For this review, use the dimensioned drawing (mm, ordinates from the lowest corner) and the shaded views. Coordinates: 2 decimals unless noted, no trailing zeros. Order: outer loops, then holes, each group sorted by start corner. A loop starts at its lowest first (then second) coordinate and runs counter-clockwise, first axis right, second up. Notation, with made-up numbers: (8.25, -30.5) -> (24.25, -30.5) arc R10 cw to (24.25, -21.5) -> close; hole circle Ø3 at (50, 62.5). An arc over 180 degrees is marked (long way). Use one line per item in the form item = value. Start each with the question number.
(1) Take a section at C-C (x = 26.5). State the section outline as (y, z) points.
(2) Take a section at A-A (z = 89). State the section outline as (x, y) points, then the cut area to 3 significant figures.
(3) Wall thickness on line 1 along X through (y, z) = (1.4, 11); line 2 along Z through (x, y) = (13, 1.85): over which ranges is each line inside the solid? List them lowest first.
(4) Insertion check: pin 1 Ø2.5 at (x, y) = (40.5, 2) entering from -Z; pin 2 Ø5 at (x, z) = (42, 34.5) entering from +Y. Each pin has a flat end and moves straight along its axis. Give the tip position at first contact, or say it passes through.
(5) Take a section at B-B (y = 1.3). State the section outline as (x, z) points.
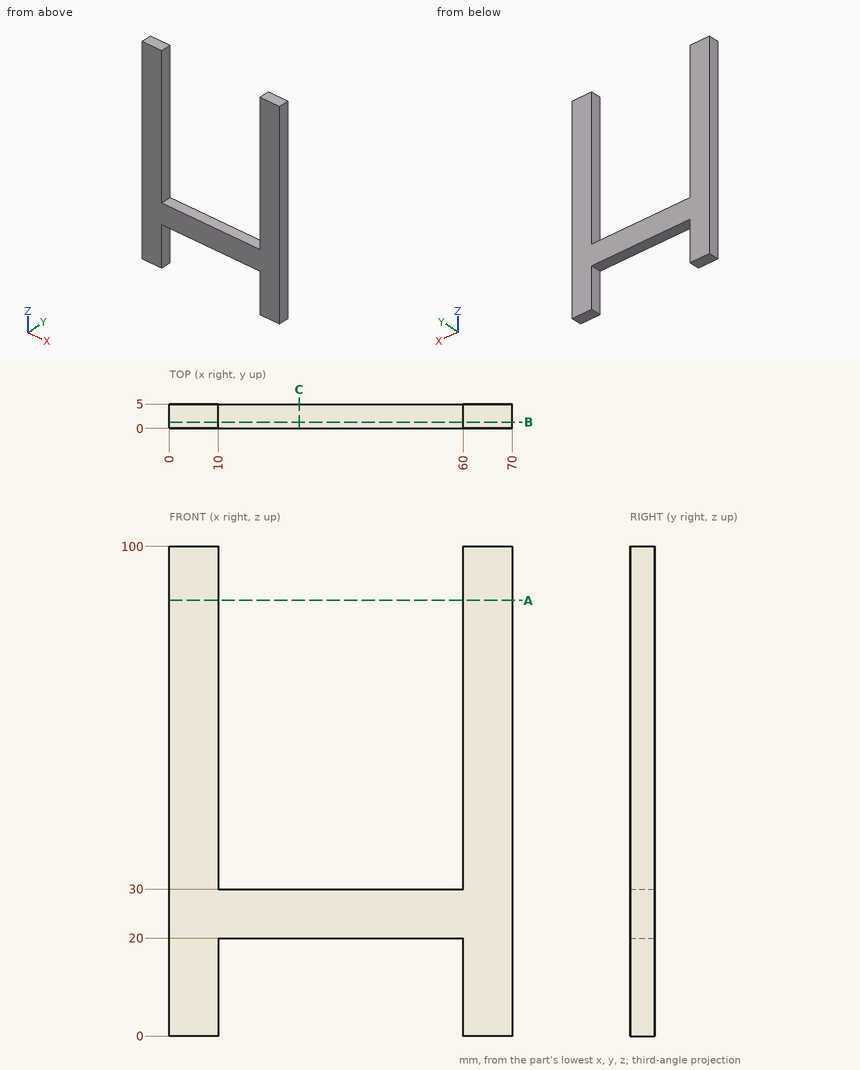
Findings:
q1.outline = (0, 20) -> (5, 20) -> (5, 30) -> (0, 30) -> close
q2.outline = (0, 0) -> (10, 0) -> (10, 5) -> (0, 5) -> close; (60, 0) -> (70, 0) -> (70, 5) -> (60, 5) -> close
q2.area = 100 mm²
q3.line_1 = 0 to 10, 60 to 70
q3.line_2 = 20 to 30
q4.pin_1 = 20
q4.pin_2 = through
q5.outline = (0, 0) -> (10, 0) -> (10, 20) -> (60, 20) -> (60, 0) -> (70, 0) -> (70, 100) -> (60, 100) -> (60, 30) -> (10, 30) -> (10, 100) -> (0, 100) -> close
